from build123d import *

# Parameters (mm, degrees)
PAD_DEPTH = 150


with BuildPart() as part:
    # Sketch → Pad (new body)
    with BuildSketch(Plane.XZ):
        Polygon((0, 72.009016), (90, 72.009016), (90, 60.009016), (50, 60.009016), (50, 9.009016), (90, 9.009016), (90, -2.990984), (0, -2.990984), (0, 9.009016), (40, 9.009016), (40, 60.009016), (0, 60.009016), align=None)
    extrude(amount=PAD_DEPTH)


solid = part.part
Source: CAD feature listing. Evaluate the final solid. Frame: model axes, mm. A direction names the side the tool comes from. Give positions to 0.01 mm unless a question says otherwise; leave off trailing zeros. Write each loop counter-clockwise with the first axis right and the second up, starting at its lowest first coordinate (ties: lowest second). Pieces come first, ordered by that corner, then holes. Notation, with made-up numbers: M 5,68 L 9,68 A14 ccw 9,95 Z; hole C -31,80.5 d9. An arc over 180 degrees is marked long. Answer as a JSON object with one key per item and string values.
Q1. Cut plane C-C, the plane z = 25. Return the cut outline in (x, y).
Geometry check:
{"outline": "M 40,-150 L 50,-150 L 50,0 L 40,0 Z"}
Q2. Mould query, pull axis Z, two halves, no side actions, for faces 4 (the face through (44, -74, 72.009)), 5 (the face through (90, -74, 3)), 6 (the face through (70, -74, 9.009)). Classes: +Z half, -Z half, draft (parallel to the pull), parting line (faces both ways), or undercut.
Geometry check:
{"face 4": "+Z half", "face 5": "draft", "face 6": "undercut"}
Q3. Cut plane A-A, the plane x = 59. Return the cut outline in (y, z).
Geometry check:
{"outline": "M -150,-2.99 L 0,-2.99 L 0,9.01 L -150,9.01 Z; M -150,60.01 L 0,60.01 L 0,72.01 L -150,72.01 Z"}
Q4. Contact query for flat-ended pins moving along their axis: P1, Ø6, axis at x = 35, z = 15.5, coming from the +Y side; P2, Ø2, axis at y = -90.5, z = 55.5, coming from the -X side; P3, Ø15.5, axis at y = -42.5, z = 23.5, coming from the +X side. Output: stop coordinate, or through.
Geometry check:
{"P1": "passes through", "P2": "stops at x = 40", "P3": "stops at x = 50"}
Q5. Cut plane B-B, the plane y = -116. Return the cut outline in (x, z), then the cut area to 3 significant figures.
Geometry check:
{"outline": "M 0,-2.99 L 90,-2.99 L 90,9.01 L 50,9.01 L 50,60.01 L 90,60.01 L 90,72.01 L 0,72.01 L 0,60.01 L 40,60.01 L 40,9.01 L 0,9.01 Z", "area": "2,670 mm^2"}
Q6. Ray query, line 1 along Z through (x, y) = (68.5, -68); line 2 along X through (y, z) = (-125, 29.5). Return the intervals inside material, ascending.
Geometry check:
{"line 1": "z = -2.99 to 9.01, 60.01 to 72.01", "line 2": "x = 40 to 50"}
Q7. Access query for faces 1 (the face through (0, -74, 3)), 2 (the face through (70, -74, 60.009)), 3 (the face through (20, -74, 9.009)). Directions: +Z, -Z, +X, -X, +Y, -Y. A direction counts if a zero-diameter tool reaches every point of the face in a straight line with its end or side. Return the directions, or none.
Geometry check:
{"face 1": "+Z, -Z, -X, +Y, -Y", "face 2": "+X, +Y, -Y", "face 3": "-X, +Y, -Y"}
